Source: CAD feature listing. Evaluate the final solid. Frame: model axes, mm. A direction names the side the tool comes from. Give positions to 0.01 mm unless a question says otherwise; leave off trailing zeros. Order: outer loops, then holes, each group sorted by start corner. A loop starts at its lowest first (then second) coordinate and runs counter-clockwise, first axis right, second up. Notation, with made-up numbers: (67.5, -35) -> (100.5, -35) arc R18 cw to (100.5, -25) -> close; hole circle Ø3 at (29, 50). An arc over 180 degrees is marked (long way). Use CSV: the item, a comma, the result in double quotes.
```python
from build123d import *

# Parameters (mm, degrees)
SKETCH_1_W          = 94.97478029
SKETCH_1_H          = 42.97467615
SKETCH_1_W_2        = 90.97478029
SKETCH_1_H_2        = 38.97467615
EXTRUDE_1_DEPTH     = 13.5
SKETCH_2_W          = 9
SKETCH_2_H          = 9
EXTRUDE_2_DEPTH     = 13.5
SKETCH_3_R          = 1.6
CUT_EXTRUDE_1_DEPTH = 13.5
SKETCH_4_W          = 2
SKETCH_4_H          = 16.5
CUT_EXTRUDE_2_DEPTH = 8.8
FILLET_1_R          = 5
FILLET_2_R          = 0.6
SKETCH_5_W          = 4
SKETCH_5_H          = 6.600000242
CUT_EXTRUDE_3_DEPTH = 2
FILLET_3_R          = 1
SKETCH_6_W          = 6.428772381
SKETCH_6_H          = 3.6
SKETCH_6_W_2        = 9.94
SKETCH_6_H_2        = 3.75999995
CUT_EXTRUDE_4_DEPTH = 2
FILLET_4_R          = 0.5
CHAMFER_1_SIZE      = 1
CHAMFER_1_SIZE2     = 1.428148007
FILLET_5_R          = 5
CHAMFER_2_SIZE      = 0.8


with BuildPart() as part:
    # 草图1 → 凸台-拉伸1 (new body)
    with BuildSketch(Plane.XY.offset(1.6000508)):
        with Locations((45.00009017, -19.0000381)):
            Rectangle(SKETCH_1_W, SKETCH_1_H)
        with Locations((45.00009017, -19.0000381)):
            Rectangle(SKETCH_1_W_2, SKETCH_1_H_2, mode=Mode.SUBTRACT)
    extrude(amount=EXTRUDE_1_DEPTH)

    # 草图2 → 凸台-拉伸2 (add)
    with BuildSketch(Plane.XY.offset(1.6000508)):
        with Locations((4.012700025, -4.012700025)):
            Rectangle(SKETCH_2_W, SKETCH_2_H)
        with Locations((85.987480315, -4.012700025)):
            Rectangle(SKETCH_2_W, SKETCH_2_H)
        with Locations((4.012700025, -33.987376175)):
            Rectangle(SKETCH_2_W, SKETCH_2_H)
        with Locations((85.987480315, -33.987376175)):
            Rectangle(SKETCH_2_W, SKETCH_2_H)
    extrude(amount=EXTRUDE_2_DEPTH)

    # 草图3 → 切除-拉伸1 (cut)
    with BuildSketch(Plane.XY.offset(1.6000508)):
        with Locations((4.00000762, -4.00000762)):
            Circle(SKETCH_3_R)
        with Locations((86.00017272, -4.00000762)):
            Circle(SKETCH_3_R)
        with Locations((86.00017272, -34.00006858)):
            Circle(SKETCH_3_R)
        with Locations((4.00000762, -34.00006858)):
            Circle(SKETCH_3_R)
    extrude(amount=CUT_EXTRUDE_1_DEPTH, mode=Mode.SUBTRACT)

    # 草图4 → 切除-拉伸2 (cut)
    with BuildSketch(Plane.XY.offset(1.6000508)):
        with Locations((-1.487299975, -18.9999873)):
            Rectangle(SKETCH_4_W, SKETCH_4_H)
        with Locations((91.487480315, -18.939077978)):
            Rectangle(SKETCH_4_W, SKETCH_4_H)
    extrude(amount=CUT_EXTRUDE_2_DEPTH, mode=Mode.SUBTRACT)

    # 圆角1
    fillet_1_edges = [part.edges().sort_by_distance(p)[0] for p in [
        (81.487480315, -8.512700025, 8.3500508),
        (8.512700025, -29.487376175, 8.3500508),
        (81.487480315, -29.487376175, 8.3500508),
        (8.512700025, -8.512700025, 8.3500508),
    ]]
    fillet(fillet_1_edges, radius=FILLET_1_R)

    # 圆角2
    fillet_2_edges = [part.edges().sort_by_distance(p)[0] for p in [
        (-1.487299975, -27.2499873, 10.4000508),
        (-1.487299975, -10.7499873, 10.4000508),
        (91.487480315, -27.189077978, 10.4000508),
        (91.487480315, -10.689077978, 10.4000508),
    ]]
    fillet(fillet_2_edges, radius=FILLET_2_R)

    # 草图5 → 切除-拉伸3 (cut)
    with BuildSketch(Plane(origin=(0, 2.487299975, 0), x_dir=(1, 0, 0), z_dir=(0, 1, 0))):
        with Locations((30.00006096, -11.800050679)):
            Rectangle(SKETCH_5_W, SKETCH_5_H)
        with Locations((60.00011938, -11.800050679)):
            Rectangle(SKETCH_5_W, SKETCH_5_H)
    extrude(amount=-CUT_EXTRUDE_3_DEPTH, mode=Mode.SUBTRACT)

    # 圆角3
    fillet_3_edges = [part.edges().sort_by_distance(p)[0] for p in [
        (28.00006096, 1.487299975, 8.500050558),
        (32.00006096, 1.487299975, 8.500050558),
        (58.00011938, 1.487299975, 8.500050558),
        (62.00011938, 1.487299975, 8.500050558),
    ]]
    fillet(fillet_3_edges, radius=FILLET_3_R)

    # 草图6 → 切除-拉伸4 (cut)
    with BuildSketch(Plane.XZ.offset(40.487376175)):
        with Locations((71.78078399, 13.3000508)):
            Rectangle(SKETCH_6_W, SKETCH_6_H)
        with Locations((57.0001143, 13.220050825)):
            Rectangle(SKETCH_6_W_2, SKETCH_6_H_2)
    extrude(amount=-CUT_EXTRUDE_4_DEPTH, mode=Mode.SUBTRACT)

    # 圆角4
    fillet_4_edges = [part.edges().sort_by_distance(p)[0] for p in [
        (52.0301143, -39.487376175, 11.34005085),
        (61.9701143, -39.487376175, 11.34005085),
    ]]
    fillet(fillet_4_edges, radius=FILLET_4_R)

    # 倒角1
    chamfer_1_edges = [part.edges().sort_by_distance(p)[0] for p in [
        (52.0301143, -40.487376175, 13.470050825),
        (57.0001143, -40.487376175, 11.34005085),
        (61.9701143, -40.487376175, 13.470050825),
        (52.17656091, -40.487376175, 11.48649746),
        (61.823667691, -40.487376175, 11.48649746),
    ]]
    chamfer_1_side = [part.faces().sort_by_distance(p)[0] for p in [
        (44.12674601, -40.487376175, 8.107577696),
    ]]
    chamfer(chamfer_1_edges, length=CHAMFER_1_SIZE, length2=CHAMFER_1_SIZE2, reference=chamfer_1_side[0])

    # 圆角5
    fillet_5_edges = [part.edges().sort_by_distance(p)[0] for p in [
        (-2.487299975, 2.487299975, 8.3500508),
        (92.487480315, 2.487299975, 8.3500508),
        (92.487480315, -40.487376175, 8.3500508),
        (-2.487299975, -40.487376175, 8.3500508),
    ]]
    fillet(fillet_5_edges, radius=FILLET_5_R)

    # 倒角2
    chamfer_2_edges = [part.edges().sort_by_distance(p)[0] for p in [
        (92.487480315, -27.189077978, 5.7000508),
        (92.487480315, -18.939077978, 10.4000508),
        (92.487480315, -10.689077978, 5.7000508),
        (92.487480315, -27.013342047, 10.224314869),
        (92.487480315, -10.864813909, 10.224314869),
    ]]
    chamfer(chamfer_2_edges, length=CHAMFER_2_SIZE)


solid = part.part
```
1. Ray query, line 1 along X through (y, z) = (-29, 3.5); line 2 along Y through (x, z) = (27, 7.5); line 3 along X through (y, z) = (-3, 13.75). Return the intervals inside material, ascending.
Answer below:
line 1,"x = -2.49 to -0.49, 90.49 to 92.49"
line 2,"y = -40.49 to -38.49, 0.49 to 2.49"
line 3,"x = -2.49 to 2.75, 5.25 to 8.51, 81.49 to 84.75, 87.25 to 92.49"
2. Mould query, pull axis X, two halves, no side actions, for faces 1 (the cylindrical face through (82.913, -30.991, 8.445)), 2 (the flat face through (30, 2, 8.5)), 3 (the flat face through (-2, -10.75, 6)), 4 (the cylindrical face through (-1.061, 0.984, 8.445)). Classes: released by +X, released by -X, zero draft, split by the parting line, or undercut.
Answer below:
face 1,"undercut"
face 2,"undercut"
face 3,"zero draft"
face 4,"released by -X"
3. Section query D-D on z = 4.25. Count the separate pieces of the cut face and the enclosed holes in it, plus the area to 3 significant figures.
Answer below:
separate pieces,"2"
enclosed holes,"4"
area,"718 mm²"
4. Section query A-A on y = -18. Return loops of the section in (x, z), plus the area to 3 significant figures.
Answer below:
outline,"(-2.49, 10.4) -> (-0.49, 10.4) -> (-0.49, 15.1) -> (-2.49, 15.1) -> close; (90.49, 10.4) -> (91.69, 10.4) -> (92.49, 11.2) -> (92.49, 15.1) -> (90.49, 15.1) -> close"
area,"18.5 mm²"
5. Access query for faces 5 (the flat face through (45, 1, 1.6)), 6 (the flat face through (-2, -19, 10.4)), 7 (the flat face through (62, 2, 12)), 8 (the flat face through (45, 2, 15.1)), 9 (the cylindrical face through (7.009, -30.913, 8.445)). Directions: +Z, -Z, +X, -X, +Y, -Y. A direction counts if a zero-diameter tool reaches every point of the face in a straight line with its end or side. Return the directions, or none.
Answer below:
face 5,"-Z, +X, -X, +Y, -Y"
face 6,"-Z, +X, -X"
face 7,"+Z, +Y"
face 8,"+Z, +X, -X, +Y, -Y"
face 9,"+Z, -Z"
6. Section query B-B on x = 49.5. Return loops of the section in (y, z).
Answer below:
outline,"(-40.49, 1.6) -> (-38.49, 1.6) -> (-38.49, 15.1) -> (-40.49, 15.1) -> close; (0.49, 1.6) -> (2.49, 1.6) -> (2.49, 15.1) -> (0.49, 15.1) -> close"
7. Pin query (flat end, axial travel): P1, Ø2, axis at y = 2, z = 12.5, coming from the +X side; P2, Ø0.6, axis at y = 2, z = 12.5, coming from the -X side; P3, Ø3.5, axis at x = 4, y = -34, coming from the +Z side; P4, Ø1, axis at x = 30.5, y = 1, coming from the +Z side. Return the tip coordinate at first contact, or that it passes through.
Answer below:
P1,"stops at x = 91.05"
P2,"stops at x = -0.18"
P3,"stops at z = 15.1"
P4,"stops at z = 8.5"
8. Section query C-C on x = 4.5. Return loops of the section in (y, z), plus the area to 3 significant figures.
Answer below:
outline,"(-40.49, 1.6) -> (-35.52, 1.6) -> (-35.52, 15.1) -> (-40.49, 15.1) -> close; (-32.48, 1.6) -> (-29.59, 1.6) -> (-29.59, 15.1) -> (-32.48, 15.1) -> close; (-8.41, 1.6) -> (-5.52, 1.6) -> (-5.52, 15.1) -> (-8.41, 15.1) -> close; (-2.48, 1.6) -> (2.49, 1.6) -> (2.49, 15.1) -> (-2.48, 15.1) -> close"
area,"212 mm²"
